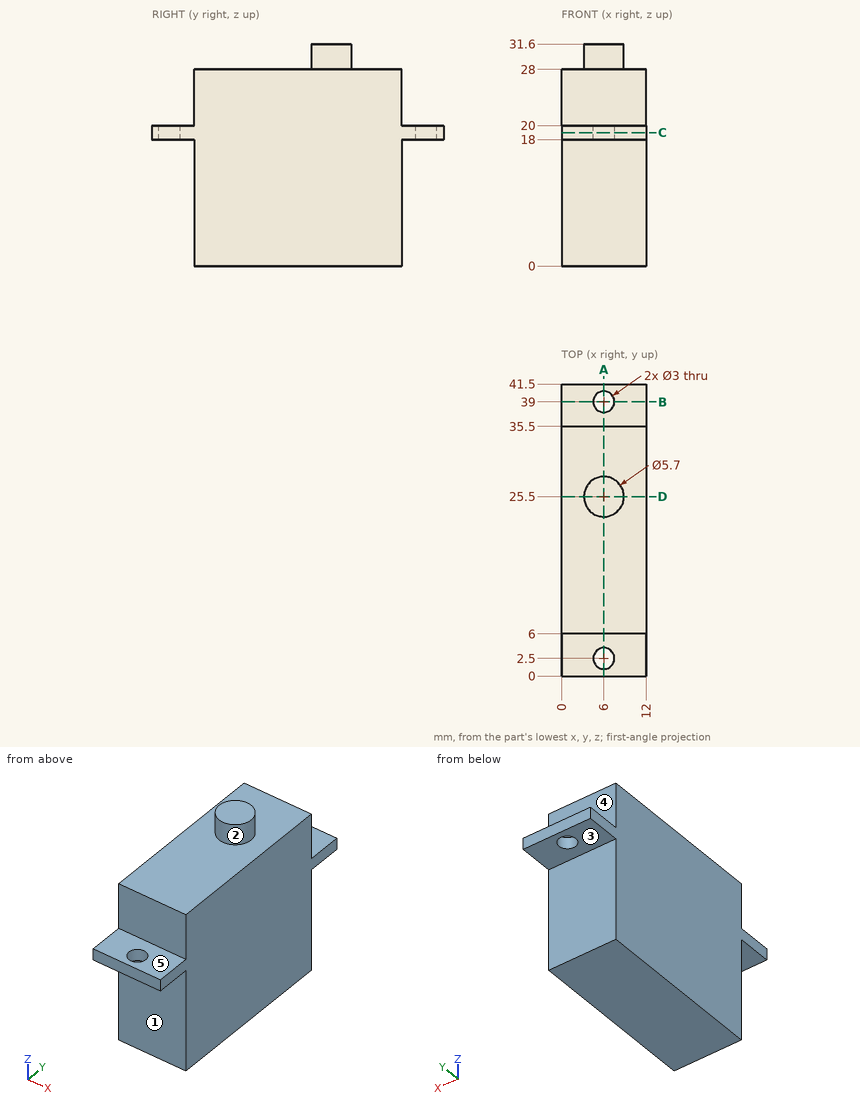
Can you work these out from the drawing? Everything is in mm from the part's minimum corner. A direction names the side the tool comes from. Coordinates: 2 decimals unless noted, no trailing zeros. Loops run counter-clockwise (first coordinate to the right, second up) from the corner with the lowest first, then second, coordinate; pieces in that order, holes last. Notation, with made-up numbers: (39, 32.25) -> (88, 32.25) arc R22 cw to (88, 62.25) -> close; hole circle Ø6 at (-21, 68.25). An arc over 180 degrees is marked (long way). Return JSON: item names as keys, results as strings.
1) If we section it at A-A, the plane x = 6: Write out the boundary of the cut face in (y, z).
Results below:
{"outline": "(0, 18) -> (1, 18) -> (1, 20) -> (0, 20) -> close; (4, 18) -> (6, 18) -> (6, 0) -> (35.5, 0) -> (35.5, 18) -> (37.5, 18) -> (37.5, 20) -> (35.5, 20) -> (35.5, 28) -> (28.35, 28) -> (28.35, 31.6) -> (22.65, 31.6) -> (22.65, 28) -> (6, 28) -> (6, 20) -> (4, 20) -> close; (40.5, 18) -> (41.5, 18) -> (41.5, 20) -> (40.5, 20) -> close"}
2) If we section it at B-B, the plane y = 39: Write out the boundary of the cut face in (x, z), then the cut area to 3 significant figures.
Results below:
{"outline": "(0, 18) -> (4.5, 18) -> (4.5, 20) -> (0, 20) -> close; (7.5, 18) -> (12, 18) -> (12, 20) -> (7.5, 20) -> close", "area": "18.0 mm²"}
3) If we section it at D-D, the plane y = 25.5: Write out the boundary of the cut face in (x, z).
Results below:
{"outline": "(0, 0) -> (12, 0) -> (12, 28) -> (8.85, 28) -> (8.85, 31.6) -> (3.15, 31.6) -> (3.15, 28) -> (0, 28) -> close"}
4) If we section it at C-C, the plane z = 19: Write out the boundary of the cut face in (x, y).
Results below:
{"outline": "(0, 0) -> (12, 0) -> (12, 41.5) -> (0, 41.5) -> close; hole circle Ø3 at (6, 2.5); hole circle Ø3 at (6, 39)"}
5) For the marked faces 1, 2, 3, 4 and 5, which set-ups out of +Z, -Z, +X, -X, +Y, -Y let a thin tool reach every point of the face, with its end or its side?
Results below:
{"face 1": "-Z, +X, -X, -Y", "face 2": "+Z", "face 3": "-Z, +X, -X, +Y", "face 4": "+Z, +X, -X, +Y", "face 5": "+Z, +X, -X, -Y"}
6) I need wall thicknesses on line 1 (Y direction, x = 6, z = 19.25); line 2 (Z direction, x = 4.75, y = 20); line 3 (Z direction, x = 10.5, y = 3). Which ranges of each line are inside material? Lowest first, please. Write a range as from..to.
Results below:
{"line 1": "0..1, 4..37.5, 40.5..41.5", "line 2": "0..28", "line 3": "18..20"}
7) Will these pins go through, and if not, where does the flat tip stop? pin 1 (4 mm diameter, centred on y = 35, z = 22, fed in from -X); pin 2 (5 mm diameter, centred on x = 6, y = 2.5, fed in from +Z); pin 3 (3.5 mm diameter, centred on x = 7.5, z = 7.5, fed in from -Y); pin 4 (6 mm diameter, centred on x = 3.5, z = 5, fed in from +Y).
Results below:
{"pin 1": "x = 0", "pin 2": "z = 20", "pin 3": "y = 6", "pin 4": "y = 35.5"}
